Geometry check sheet. Reference: the model listing, model coordinates, mm. A direction names the side the tool comes from. Round coordinates to 2 decimals unless told otherwise and drop trailing zeros. Write each loop counter-clockwise with the first axis right and the second up, starting at its lowest first coordinate (ties: lowest second). Pieces come first, ordered by that corner, then holes. Notation, with made-up numbers: (48.25, 10) -> (79.25, 10) arc R13 cw to (79.25, 23) -> close; hole circle Ø11 at (29, 52.25). An arc over 180 degrees is marked (long way). Put each result on its own line as item: value. Start each with the question number.
from build123d import *

# Parameters (mm, degrees)
BOSS_EXTRU_1_DEPTH      = 10
BOSS_EXTRU_3_START      = 2
BOSS_EXTRU_3_DEPTH      = 2
BOSS_EXTRU_4_DEPTH      = 2
ENL_V_MAT_EXTRU_2_DEPTH = 2
ENL_V_MAT_EXTRU_3_DEPTH = 2
CHANFREIN1_SIZE         = 2


with BuildPart() as part:
    # Esquisse1 → Boss.-Extru.1 (new body)
    with BuildSketch(Plane(origin=(0, 0, 0), x_dir=(0, 1, 0), z_dir=(0, 0, 1))):
        with BuildLine():
            Line((-7.89, -21.71), (-7.89, 21.71))
            ThreePointArc((-7.89, 21.71), (0, 29.6), (7.89, 21.71))
            Line((7.89, 21.71), (7.89, -21.71))
            ThreePointArc((7.89, -21.71), (0, -29.6), (-7.89, -21.71))
        make_face()
        Polygon((-1.968764418, -18.3), (-3.937528836, -21.71), (-1.968764418, -25.12), (1.968764418, -25.12), (3.937528836, -21.71), (1.968764418, -18.3), align=None, mode=Mode.SUBTRACT)
        Polygon((1.968764418, 18.3), (-1.968764418, 18.3), (-3.937528836, 21.71), (-1.968764418, 25.12), (1.968764418, 25.12), (3.937528836, 21.71), align=None, mode=Mode.SUBTRACT)
    extrude(amount=BOSS_EXTRU_1_DEPTH)

    # Esquisse3 → Boss.-Extru.3 (add)
    with BuildSketch(Plane(origin=(0, 0, 0), x_dir=(1, 0, 0), z_dir=(0, 0, -1)).offset(BOSS_EXTRU_3_START)):
        with BuildLine():
            ThreePointArc((21.71, -7.89), (27.289072504, -5.579072504), (29.6, 0))
            ThreePointArc((29.6, 0), (27.289072504, 5.579072504), (21.71, 7.89))
            ThreePointArc((21.71, 7.89), (13.82, 0), (21.71, -7.89))
        make_face()
        Polygon((21.71, -3.937528836), (18.3, -1.968764418), (18.3, 1.968764418), (21.71, 3.937528836), (25.12, 1.968764418), (25.12, -1.968764418), align=None, mode=Mode.SUBTRACT)
    extrude(amount=-BOSS_EXTRU_3_DEPTH)

    # Esquisse4 → Boss.-Extru.4 (add)
    with BuildSketch(Plane.XY.offset(10)):
        with BuildLine():
            ThreePointArc((-21.71, -7.89), (-16.130927496, -5.579072504), (-13.82, 0))
            ThreePointArc((-13.82, 0), (-16.130927496, 5.579072504), (-21.71, 7.89))
            ThreePointArc((-21.71, 7.89), (-29.6, 0), (-21.71, -7.89))
        make_face()
        Polygon((-25.12, -1.968764418), (-25.12, 1.968764418), (-21.71, 3.937528836), (-18.3, 1.968764418), (-18.3, -1.968764418), (-21.71, -3.937528836), align=None, mode=Mode.SUBTRACT)
    extrude(amount=BOSS_EXTRU_4_DEPTH)

    # Esquisse5 → Enlèv. mat.-Extru.2 (cut)
    with BuildSketch(Plane(origin=(0, 0, 0), x_dir=(1, 0, 0), z_dir=(0, 0, -1))):
        Polygon((-16.3, -3.123464956), (-16.3, 3.123464956), (-21.71, 6.246929913), (-27.12, 3.123464956), (-27.12, -3.123464956), (-21.71, -6.246929913), align=None)
    extrude(amount=-ENL_V_MAT_EXTRU_2_DEPTH, mode=Mode.SUBTRACT)

    # Esquisse6 → Enlèv. mat.-Extru.3 (cut)
    with BuildSketch(Plane.XY.offset(10)):
        Polygon((27.12, -3.123464956), (27.12, 3.123464956), (21.71, 6.246929913), (16.3, 3.123464956), (16.3, -3.123464956), (21.71, -6.246929913), align=None)
    extrude(amount=-ENL_V_MAT_EXTRU_3_DEPTH, mode=Mode.SUBTRACT)

    # Chanfrein1
    chanfrein1_edges = [part.edges().sort_by_distance(p)[0] for p in [
        (20.005, 2.953146627, -2),
        (18.3, 0, -2),
        (20.005, -2.953146627, -2),
        (23.415, -2.953146627, -2),
        (25.12, 0, -2),
        (23.415, 2.953146627, -2),
        (-25.12, 0, 12),
        (-23.415, 2.953146627, 12),
        (-20.005, 2.953146627, 12),
        (-18.3, 0, 12),
        (-20.005, -2.953146627, 12),
        (-23.415, -2.953146627, 12),
    ]]
    chamfer(chanfrein1_edges, length=CHANFREIN1_SIZE - 0.0001)  # a hair under: the kernel refuses the full size


solid = part.part
(1) Go/stop test with flat-tipped pins: pin 1 Ø8 at (x, y) = (-10.5, 4) entering from -Z; pin 2 Ø5.5 at (x, y) = (19.5, 1.5) entering from +Z; pin 3 Ø4 at (y, z) = (4, 3.5) entering from +X. Record where each tip stops, or that it passes through.
(2) Sectioned sample at C-C (x = 0.5). Record the cut outline in (y, z), and give its area (3 significant figures).
(3) Sectioned sample at B-B (y = 4.5). Record the cut outline in (x, z), and give its area (3 significant figures).
(4) Mould release check, pull along Y, two halves, no side actions. Record for faces 4 (the flat face through (0, -7.89, 5)), 5 (the flat face through (19.47, -3.79, -0.99)): +Y half, -Y half, draft (parallel to the pull), parting line (faces both ways), or undercut.
(5) Material ranges on L1, parallel to X at y = -1, z = 5.5; L2, parallel to X at y = -2.75, z = 0.25; L3, parallel to Z at x = 9, y = 6.75, recorded low to high. Write a range as from..to.
(6) Sectioned sample at A-A (z = 3). Record the cut outline in (x, y).
(7) Sectioned sample at D-D (y = -7). Record the cut outline in (x, z).
(8) Set-up check for faces 1 (the flat face through (-18.3, 0, 6)), 2 (the flat face through (-24.453, 4.663, 0.986)), 3 (the flat face through (19, -3, 8)): record each of +Z, -Z, +X, -X, +Y, -Y from which the full face is reachable in a straight line by a thin tool's end or side.
Found:
1. pin 1: z = 0
1. pin 2: z = 8
1. pin 3: x = 29.34
2. outline: (-7.89, 0) -> (7.89, 0) -> (7.89, 10) -> (-7.89, 10) -> close
2. area: 158 mm2
3. outline: (-28.19, 0) -> (-24.74, 0) -> (-24.74, 2) -> (-18.68, 2) -> (-18.68, 0) -> (15.23, 0) -> (15.23, -2) -> (18.68, -2) -> (21.71, -0.49) -> (24.74, -2) -> (28.19, -2) -> (28.19, 10) -> (24.74, 10) -> (24.74, 8) -> (18.68, 8) -> (18.68, 10) -> (-15.23, 10) -> (-15.23, 12) -> (-18.68, 12) -> (-21.71, 10.49) -> (-24.74, 12) -> (-28.19, 12) -> close
3. area: 582 mm2
4. face 4: -Y half
4. face 5: undercut
5. L1: -29.54..-25.12, -18.3..18.3, 25.12..29.54
5. L2: -29.11..-27.12, -16.3..19.65, 23.77..29.11
5. L3: 0..10
6. outline: (-21.71, -7.89) -> (21.71, -7.89) arc R7.89 ccw to (21.71, 7.89) -> (-21.71, 7.89) arc R7.89 ccw to start; hole (-25.12, -1.97) -> (-21.71, -3.94) -> (-18.3, -1.97) -> (-18.3, 1.97) -> (-21.71, 3.94) -> (-25.12, 1.97) -> close; hole (18.3, -1.97) -> (21.71, -3.94) -> (25.12, -1.97) -> (25.12, 1.97) -> (21.71, 3.94) -> (18.3, 1.97) -> close
7. outline: (-25.35, 0) -> (18.07, 0) -> (18.07, -2) -> (25.35, -2) -> (25.35, 10) -> (-18.07, 10) -> (-18.07, 12) -> (-25.35, 12) -> close
8. face 1: +Z, -Z
8. face 2: -Z
8. face 3: +Z
